Autodesk Inventor part; units mm, degrees
ref_plane "YZ Plane" through (0, 0, 0) normal (1, 0, 0) x (0, 1, 0)
ref_plane "XZ Plane" through (0, 0, 0) normal (0, 1, 0) x (-1, 0, 0)
ref_plane "XY Plane" through (0, 0, 0) normal (0, 0, 1) x (1, 0, 0)
sketch "草圖1" plane through (0, 0, 0) normal (0, 0, 1) x (1, 0, 0)
  circle A0 centre (0, 0) radius 7.5
  line L0 (5.95, -1.45) -> (-5.95, -1.45)
  line L1 (-5.95, -1.45) -> (-5.95, 1.45)
  line L2 (-5.95, 1.45) -> (5.95, 1.45)
  line L3 (5.95, 1.45) -> (5.95, -1.45)
  line L4 (5.95, -1.45) -> (-5.95, 1.45) construction
  line L5 (-5.95, -1.45) -> (5.95, 1.45) construction
  line L6 (1.45, -5.95) -> (-1.45, -5.95)
  line L7 (-1.45, -5.95) -> (-1.45, 5.95)
  line L8 (-1.45, 5.95) -> (1.45, 5.95)
  line L9 (1.45, 5.95) -> (1.45, -5.95)
  line L10 (1.45, -5.95) -> (-1.45, 5.95) construction
  line L11 (-1.45, -5.95) -> (1.45, 5.95) construction
  point P0 (-1.45, 1.45)
  point P1 (1.45, 1.45)
  point P2 (1.45, -1.45)
  point P3 (-1.45, -1.45)
  dimension "d0" = 15
  dimension "d1" = 11.9
  dimension "d2" = 2.9
extrude "擠出1" add sketch "草圖1" along normal blind 3
properties part number "rod_7"
Read the model definition and answer for the solid it produces. Units are mm, in the model's axes. A direction names the side the tool comes from. Coordinates: 2 decimals unless noted, no trailing zeros. Loops run counter-clockwise (first coordinate to the right, second up) from the corner with the lowest first, then second, coordinate; pieces in that order, holes last.
Q1. The mould has two halves that part along X. Classify faces 3 (the face through (2, -2, 3)), 4 (the face through (4, 1.45, 1)), 5 (the face through (-7.493, -0.33, 1.479)): +X half, -X half, draft (parallel to the pull), parting line (faces both ways), or undercut.
Q2. Which of the six approach directions +Z, -Z, +X, -X, +Y, -Y give full straight-line access (tool end or side, diameter ignored) to faces 1 (the face through (1.45, -4, 1)), 2 (the face through (2, -2, 0))?
Q3. Consider probe 1 along Y at (x, z) = (0, 0.35); probe 2 along Y at (x, z) = (-2, 0.2). Determine where each line is inside the solid, lowest interval first.
Q4. The part is cut by section C-C on z = 0.3. Write down the section's boundary in (x, y), and give its area (3 significant figures).
Q5. The part is cut by section A-A on y = 0. Write down the section's boundary in (x, z).
Q6. Each of these flat-tipped pins is pushed along its axis until it touches: pin 1 Ø1.5 at (y, z) = (-4.5, 1) entering from +X; pin 2 Ø1.5 at (y, z) = (-1.5, 2) entering from +X; pin 3 Ø1.4 at (x, z) = (0.5, 1) entering from -Y; pin 4 Ø0.9 at (x, z) = (-4.5, 1.5) entering from +Y. Where does it stop, or does it pass through?
Results below:
1. face 3: draft
1. face 4: undercut
1. face 5: parting line
2. face 1: +Z, -Z
2. face 2: -Z, +X, -X, +Y, -Y
3. probe 1: y = -7.5 to -5.95, 5.95 to 7.5
3. probe 2: y = -7.23 to -1.45, 1.45 to 7.23
4. outline: circle Ø15 at (0, 0); hole (-5.95, -1.45) - (-1.45, -1.45) - (-1.45, -5.95) - (1.45, -5.95) - (1.45, -1.45) - (5.95, -1.45) - (5.95, 1.45) - (1.45, 1.45) - (1.45, 5.95) - (-1.45, 5.95) - (-1.45, 1.45) - (-5.95, 1.45) - close
4. area: 116 mm2
5. outline: (-7.5, 0) - (-5.95, 0) - (-5.95, 3) - (-7.5, 3) - close; (5.95, 0) - (7.5, 0) - (7.5, 3) - (5.95, 3) - close
6. pin 1: stops at x = 6.5
6. pin 2: stops at x = 7.46
6. pin 3: stops at y = -7.5
6. pin 4: stops at y = 6.31
